from build123d import *

# Parameters (mm, degrees)
SKETCH_1_W                    = 35
SKETCH_1_H                    = 5
HOLE_WIZARD_3_4_3_4_1_D       = 3.4
HOLE_WIZARD_3_4_3_4_1_DEPTH   = 5
HOLE_WIZARD_M48_1_D           = 52
HOLE_WIZARD_M48_1_DEPTH       = 5
HOLE_WIZARD_M48_1_CBORE_D     = 58.1
HOLE_WIZARD_M48_1_CBORE_DEPTH = 4
FILLET_1_R                    = 1
SKETCH_17_R                   = 2.8
CUT_EXTRUDE_9_DEPTH           = 2.7


with BuildPart() as part:
    # 草图1 → 旋转1 (revolve)
    with BuildSketch(Plane(origin=(0, 0, 0), x_dir=(1, 0, 0), z_dir=(0, 1, 0))):
        with Locations((17.5, 26.5)):
            Rectangle(SKETCH_1_W, SKETCH_1_H)
    revolve(axis=Axis((0, 0, -29), (0, 0, 1)))

    # Ø3.4 (3.4) 直径孔1
    with Locations(Plane(origin=(0, 0, -29), x_dir=(-1, 0, 0), z_dir=(0, 0, -1))):
        with Locations((0, -32), (-32, 0), (0, 32), (32, 0)):
            Hole(HOLE_WIZARD_3_4_3_4_1_D / 2, depth=HOLE_WIZARD_3_4_3_4_1_DEPTH)

    # M48 六角头螺栓的柱形沉头孔1
    with Locations(Plane.XY.offset(-24)):
        with Locations((0, 0)):
            CounterBoreHole(HOLE_WIZARD_M48_1_D / 2, HOLE_WIZARD_M48_1_CBORE_D / 2, HOLE_WIZARD_M48_1_CBORE_DEPTH, depth=HOLE_WIZARD_M48_1_DEPTH)

    # 圆角1
    fillet_1_edges = [part.edges().sort_by_distance(p)[0] for p in [
        (-35, 0, -29),
    ]]
    fillet(fillet_1_edges, radius=FILLET_1_R)

    # 草图17 → 切除-拉伸9 (cut)
    with BuildSketch(Plane(origin=(0, 0, -29), x_dir=(-1, 0, 0), z_dir=(0, 0, -1))):
        with Locations((0, -32)):
            Circle(SKETCH_17_R)
        with Locations((-32, 0)):
            Circle(SKETCH_17_R)
        with Locations((0, 32)):
            Circle(SKETCH_17_R)
        with Locations((32, 0)):
            Circle(SKETCH_17_R)
    extrude(amount=-CUT_EXTRUDE_9_DEPTH, mode=Mode.SUBTRACT)


solid = part.part
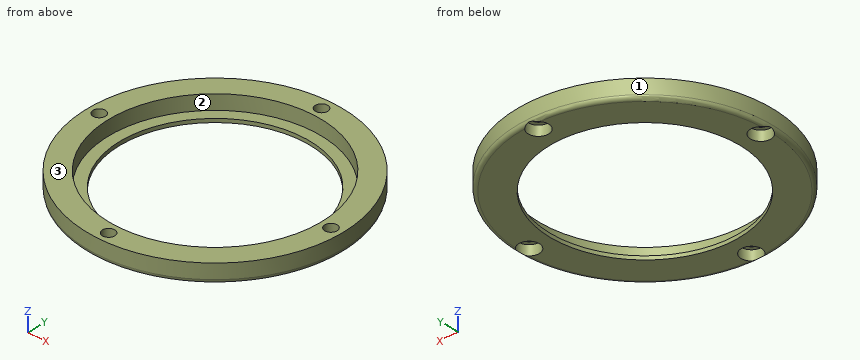
Could you check a few things on this model? Use its own coordinates, in mm. Face numbers are marked on the shaded views. Round coordinates to 2 decimals unless told otherwise and drop trailing zeros. Write each loop counter-clockwise with the first axis right and the second up, starting at its lowest first coordinate (ties: lowest second). Pieces come first, ordered by that corner, then holes. Notation, with made-up numbers: (11, 47.5) -> (53, 47.5) arc R22 cw to (53, 53.5) -> close; hole circle Ø11 at (-28.5, 19). An arc over 180 degrees is marked (long way). Use a Markdown table: item, result.
1. For pin 1 Ø2 at (y, z) = (4, -26) entering from -X; pin 2 Ø4.5 at (x, y) = (0, 32) entering from -Z; pin 3 Ø2 at (x, z) = (-6, -27.5) entering from -Y, each with a flat end and sliding along its axis, tell me the tip position at first contact or that it passes through.
Answer key:
| item | result |
|---|---|
| pin 1 | stops at x = -34.87 |
| pin 2 | stops at z = -26.3 |
| pin 3 | stops at y = -34.64 |
2. Please list where these lines run through material, in increasing order: probe 1 along Y at (x, z) = (0, -25.3); probe 2 along Y at (x, z) = (0, -27.65); probe 3 along Y at (x, z) = (-6, -26.4).
Answer key:
| item | result |
|---|---|
| probe 1 | y = -35 to -33.7, -30.3 to -29.05, 29.05 to 30.3, 33.7 to 35 |
| probe 2 | y = -35 to -34.8, -29.2 to -29.05, 29.05 to 29.2, 34.8 to 35 |
| probe 3 | y = -34.48 to -28.42, 28.42 to 34.48 |
3. If we section it at A-A (y = 0): List the corners of the cut face in (x, z) for me, then the cut area to 3 significant figures.
Answer key:
| item | result |
|---|---|
| outline | (-35, -28) arc R1 ccw to (-34.8, -28.6) -> (-34.8, -26.3) -> (-33.7, -26.3) -> (-33.7, -24) -> (-35, -24) -> close; (-30.3, -26.3) -> (-29.2, -26.3) -> (-29.2, -29) -> (-26, -29) -> (-26, -28) -> (-29.05, -28) -> (-29.05, -24) -> (-30.3, -24) -> close; (26, -29) -> (29.2, -29) -> (29.2, -26.3) -> (30.3, -26.3) -> (30.3, -24) -> (29.05, -24) -> (29.05, -28) -> (26, -28) -> close; (33.7, -26.3) -> (34.8, -26.3) -> (34.8, -28.6) arc R1 ccw to (35, -28) -> (35, -24) -> (33.7, -24) -> close |
| area | 19.5 mm^2 |
4. We'd pull the mould along X, two halves only. Please class the marked faces 1, 2 and 3: +X half, -X half, draft (parallel to the pull), parting line (faces both ways), or undercut.
Answer key:
| item | result |
|---|---|
| face 1 | parting line |
| face 2 | undercut |
| face 3 | draft |
